The model under review builds one solid part; all positions refer to its coordinate system, in mm. A direction names the side the tool comes from. Coordinates: 2 decimals unless noted, no trailing zeros. Loops run counter-clockwise (first coordinate to the right, second up) from the corner with the lowest first, then second, coordinate; pieces in that order, holes last. Notation, with made-up numbers: (49, 18) - (57, 18) arc R24 cw to (57, 31) - close; hole circle Ø11 at (86, 72.5). An arc over 180 degrees is marked (long way). Use a Markdown table: item, result. Add a question column.
1) Add section D-D, the plane x = 17.78. Give the boundary of the cut face in (y, z).
2) To check wall thickness, follow L1, parallel to Y at x = 0, z = -0.15; L2, parallel to Y at x = 18, z = -2.2; L3, parallel to X at y = -3, z = 0.8. State the ranges of each line that lie inside material, in increasing order. Write a range as [from, to].
3) Add section B-B, the plane y = 0. Give the boundary of the cut face in (x, z), and give its area (3 significant figures).
4) Add section C-C, the plane z = 0.65. Give the boundary of the cut face in (x, y).
5) Add section A-A, the plane x = 0. Give the boundary of the cut face in (y, z), and give its area (3 significant figures).
6) For faces 1 (the flat face through (0, 5, 2.667)), 2 (the flat face through (1.588, 5, 0)), list the 3-axis set-ups (+Z, -Z, +X, -X, +Y, -Y) from which the entire face can be reached by the end or side of a thin tool; tool diameter is ignored.
7) The part is to be moulded in two halves that separate along Y. For faces 3 (the cylindrical face through (-0.172, -18.555, 0.037)), 4 (the flat face through (0, 5, -2.667)), 5 (the flat face through (-1.588, 5, 0)), 6 (the cylindrical face through (-2.645, 20.147, 0.037)), say which applies: pulls with the +Y half, pulls with the -Y half, needs draft (parallel to the pull), parting line crosses it, or undercut.
8) Clearance check with flat-ended pins moving along their axes: pin 1 (1.5 mm diameter, centred on y = 5.5, z = -0.5, fed in from +X); pin 2 (1.5 mm diameter, centred on y = 13, z = -1.5, fed in from -X); pin 3 (2 mm diameter, centred on x = -2, z = 2, fed in from -Y); pin 4 (1.4 mm diameter, centred on x = 0, y = -17.78, fed in from +Z). State where each tip first meets the part, or that it passes through.
```python
from build123d import *

# Parameters (mm, degrees)
SKETCH1_R               = 20.32
SKETCH1_R_2             = 9.144
BOSS_EXTRUDE1_DEPTH     = 2.667
SKETCH2_R               = 1.4605
CUT_EXTRUDE1_DEPTH      = 30.227664224
BOSS_EXTRUDE2_START     = -2.667
BOSS_EXTRUDE2_OUTLINE_R = 9.144
BOSS_EXTRUDE2_DEPTH     = 5.334
SKETCH4_R               = 0.79375
CUT_EXTRUDE2_DEPTH      = 30.227664224


# Read off the part's stored shape, not the designer's step: Boss-Extrude2
with BuildPart() as part:
    # Sketch1 → Boss-Extrude1 (new, symmetric)
    with BuildSketch(Plane.XY):
        Circle(SKETCH1_R)
        Circle(SKETCH1_R_2, mode=Mode.SUBTRACT)
    extrude(amount=BOSS_EXTRUDE1_DEPTH, both=True)

    # Sketch2 → Cut-Extrude1 (cut, through all)
    with BuildSketch(Plane.XY.offset(2.667)):
        with Locations((12.7, 0)):
            Circle(SKETCH2_R)
        with Locations((-12.7, 0)):
            Circle(SKETCH2_R)
    extrude(amount=-CUT_EXTRUDE1_DEPTH, mode=Mode.SUBTRACT)

    # Boss-Extrude2 outline → Boss-Extrude2 (add)
    with BuildSketch(Plane.XY.offset(BOSS_EXTRUDE2_START)):
        Circle(BOSS_EXTRUDE2_OUTLINE_R)
        with BuildLine():
            Line((1.5875, 4.7625), (1.5875, 6.148361062))
            ThreePointArc((1.5875, 6.148361062), (0, -6.35), (-1.5875, 6.148361062))
            Line((-1.5875, 6.148361062), (-1.5875, 4.7625))
            Line((-1.5875, 4.7625), (1.5875, 4.7625))
        make_face(mode=Mode.SUBTRACT)
    extrude(amount=BOSS_EXTRUDE2_DEPTH)

    # Sketch4 → Cut-Extrude2 (cut, through all)
    with BuildSketch(Plane.XY.offset(2.667)):
        with Locations((0, 17.78)):
            Circle(SKETCH4_R)
        with Locations((17.78, 0)):
            Circle(SKETCH4_R)
        with Locations((0, -17.78)):
            Circle(SKETCH4_R)
        with Locations((-17.78, 0)):
            Circle(SKETCH4_R)
    extrude(amount=-CUT_EXTRUDE2_DEPTH, mode=Mode.SUBTRACT)


solid = part.part
```
From the geometry:
| question | item | result |
|---|---|---|
| 1 | outline | (-9.84, -2.67) - (-0.79, -2.67) - (-0.79, 2.67) - (-9.84, 2.67) - close; (0.79, -2.67) - (9.84, -2.67) - (9.84, 2.67) - (0.79, 2.67) - close |
| 2 | L1 | y = [-20.32, -18.57], [-16.99, -6.35], [4.76, 16.99], [18.57, 20.32] |
| 2 | L2 | y = [-9.43, -0.76], [0.76, 9.43] |
| 2 | L3 | x = [-20.1, -5.6], [5.6, 20.1] |
| 3 | outline | (-20.32, -2.67) - (-18.57, -2.67) - (-18.57, 2.67) - (-20.32, 2.67) - close; (-16.99, -2.67) - (-14.16, -2.67) - (-14.16, 2.67) - (-16.99, 2.67) - close; (-11.24, -2.67) - (-6.35, -2.67) - (-6.35, 2.67) - (-11.24, 2.67) - close; (6.35, -2.67) - (11.24, -2.67) - (11.24, 2.67) - (6.35, 2.67) - close; (14.16, -2.67) - (16.99, -2.67) - (16.99, 2.67) - (14.16, 2.67) - close; (18.57, -2.67) - (20.32, -2.67) - (20.32, 2.67) - (18.57, 2.67) - close |
| 3 | area | 101 mm^2 |
| 4 | outline | circle Ø40.64 at (0, 0); hole circle Ø1.59 at (-17.78, 0); hole circle Ø2.92 at (-12.7, 0); hole (-1.59, 4.76) - (-1.59, 6.15) arc R6.35 ccw (long way) to (1.59, 6.15) - (1.59, 4.76) - close; hole circle Ø1.59 at (0, -17.78); hole circle Ø1.59 at (0, 17.78); hole circle Ø2.92 at (12.7, 0); hole circle Ø1.59 at (17.78, 0) |
| 5 | outline | (-20.32, -2.67) - (-18.57, -2.67) - (-18.57, 2.67) - (-20.32, 2.67) - close; (-16.99, -2.67) - (-6.35, -2.67) - (-6.35, 2.67) - (-16.99, 2.67) - close; (4.76, -2.67) - (16.99, -2.67) - (16.99, 2.67) - (4.76, 2.67) - close; (18.57, -2.67) - (20.32, -2.67) - (20.32, 2.67) - (18.57, 2.67) - close |
| 5 | area | 141 mm^2 |
| 6 | face 1 | +Z, +X, -X, +Y, -Y |
| 6 | face 2 | +Z, -Z |
| 7 | face 3 | undercut |
| 7 | face 4 | needs draft |
| 7 | face 5 | undercut |
| 7 | face 6 | parting line crosses it |
| 8 | pin 1 | stops at x = 19.76 |
| 8 | pin 2 | stops at x = -16.21 |
| 8 | pin 3 | stops at y = -20.3 |
| 8 | pin 4 | passes through |
